Autodesk Inventor part; units mm, degrees
ref_plane "YZ Plane" through (0, 0, 0) normal (1, 0, 0) x (0, 1, 0)
ref_plane "XZ Plane" through (0, 0, 0) normal (0, 1, 0) x (-1, 0, 0)
ref_plane "XY Plane" through (0, 0, 0) normal (0, 0, 1) x (1, 0, 0)
sketch "スケッチ1" plane through (0, 0, 0) normal (1, 0, 0) x (0, 1, 0)
  line L0 (0, 0) -> (-96, 0)
  line L1 (-96, 0) -> (-96, -8)
  line L2 (-96, -8) -> (0, -8)
  line L3 (0, -8) -> (0, 0)
  line L4 (13, 5) -> (5, 5)
  line L5 (5, 5) -> (5, 75)
  line L6 (5, 75) -> (13, 75)
  line L7 (13, 75) -> (13, 5)
  line L8 (13, 5) -> (0, -8)
  line L9 (5, 5) -> (0, 0)
  line L10 (-44, 84) -> (13, 84)
  line L11 (13, 84) -> (13, 75)
  line L12 (-44, 76) -> (-44, 46)
  line L13 (-44, 46) -> (-36, 46)
  line L14 (-36, 46) -> (-36, 76)
  line L15 (5, 75) -> (5, 76)
  line L16 (5, 76) -> (-44, 76)
  line L17 (-44, 84) -> (-44, 76)
  point P0 (-36, 0)
  point P1 (-36, 76)
  point P2 (-44, 76)
  dimension "d0" = 8
  dimension "d2" = 8
  dimension "d3" = 70
  dimension "d4" = 96
  dimension "d17" = 13
  dimension "d36" = 8
  dimension "d37" = 41
  dimension "d53" = 1
  dimension "d54" = 8
  dimension "d55" = 30
  dimension "d72" = 57
  dimension "d86" = 30
extrude "押し出し1" add sketch "スケッチ1" along normal blind 80
sketch "スケッチ2" plane through (80, 0, 0) normal (1, 0, 0) x (0, 0, -1)
  line L0 (8, -96) -> (8, 0)
  point P0 (0, 0)
  point P1 (4, -71)
  point P2 (-50, 9)
  point P3 (-50, -40)
  dimension "d9" = 4
  dimension "d19" = 80
  dimension "d84" = 58
  dimension "d87" = 49
hole "穴1" at (80, -71, -4) at (80, 9, 50) at (80, -40, 50) direction (-1, 0, 0) diameter 2.459 depth 8.8 tip angle 118
sketch "スケッチ5" plane through (0, 13, 84) normal (0, 1, 0) x (1, 0, 0)
  line L0 (80, 8) -> (70, 8)
  line L1 (70, 8) -> (70, 30)
  line L2 (70, 30) -> (80, 30)
  line L3 (80, 30) -> (80, 8)
  line L4 (0, 0) -> (80, 0)
  line L5 (80, 79) -> (80, 0)
  point P0 (0, 84)
  dimension "d38" = 8
  dimension "d39" = 10
  dimension "d40" = 22
extrude "押し出し3" cut sketch "スケッチ5" against normal blind 80
sketch "スケッチ6" plane through (0, 13, 84) normal (0, 1, 0) x (1, 0, 0)
  line L0 (80, 8) -> (80, 0)
  line L1 (0, 0) -> (80, 0)
  point P0 (0, 84)
  point P1 (59.78, 12)
  point P2 (59.78, 26)
  dimension "d43" = 20.22
  dimension "d44" = 12
  dimension "d45" = 14
hole "穴3" at (59.78, 13, 72) at (59.78, 13, 58) direction (0, -1, 0) diameter 2.2 depth 8.8 tip angle 118
sketch "スケッチ7" plane through (0, -44, 46) normal (0, -1, 0) x (1, 0, 0)
  line L0 (80, 8) -> (80, 0)
  line L1 (80, 8) -> (70, 8)
  point P0 (0, -46)
  point P1 (67.7, 26.5)
  point P2 (67.7, 11.5)
  point P3 (52.7, 26.5)
  point P4 (52.7, 11.5)
  dimension "d58" = 15
  dimension "d59" = 15
  dimension "d60" = 12.3
  dimension "d61" = 3.5
hole "穴4" at (67.7, -44, 72.5) at (67.7, -44, 57.5) at (52.7, -44, 72.5) at (52.7, -44, 57.5) direction (0, 1, 0) diameter 2.2 depth 8 tip angle 118
sketch "スケッチ8" plane through (0, -44, 46) normal (0, -1, 0) x (1, 0, 0)
  line L0 (0, 38) -> (41.2, 38)
  line L1 (41.2, 38) -> (41.2, 8)
  line L2 (41.2, 8) -> (0, 8)
  line L3 (0, 8) -> (0, 38)
  line L4 (0, -46) -> (80, -46)
  line L5 (0, 38) -> (0, -46)
  line L6 (0, 38) -> (80, 38)
  circle A0 centre (52.7, 26.5) radius 1.1
  line L7 (80, 8) -> (70, 8)
  dimension "d75" = 11.5
  dimension "d83" = 0
extrude "押し出し4" cut sketch "スケッチ8" against normal blind 10 contours L0 L1 L2 L3
sketch "スケッチ9" plane through (0, -34, 46) normal (0, -1, 0) x (1, 0, 0)
  point P0 (0, -46)
sketch "スケッチ10" plane through (0, -34, 46) normal (0, -1, 0) x (1, 0, 0)
  line L0 (41.2, 38) -> (0, 38)
  line L1 (0, 38) -> (0, 30)
  line L2 (0, 30) -> (41.2, 30)
  line L3 (41.2, 30) -> (41.2, 38)
  line L4 (0, 38) -> (41.2, 38)
  line L5 (41.2, 38) -> (41.2, 8)
  line L6 (0, 30) -> (0, 38)
  line L7 (41.2, 30) -> (0, 30)
  point P0 (0, -46)
  point P1 (41.2, 0)
extrude "押し出し5" cut sketch "スケッチ10" against normal blind 39
sketch "スケッチ11" plane through (0, 5, 5) normal (0, -1, 0) x (1, 0, 0)
  point P0 (0, -5)
sketch "スケッチ12" plane through (0, 5, 5) normal (0, -1, 0) x (1, 0, 0)
  line L0 (41.2, 71) -> (49.2, 71)
  line L1 (49.2, 71) -> (49.2, 49)
  line L2 (49.2, 49) -> (41.2, 49)
  line L3 (41.2, 49) -> (41.2, 71)
  point P0 (0, -5)
  point P1 (70, 71)
  point P2 (41.2, 71)
  dimension "d76" = 8
  dimension "d77" = 22
extrude "押し出し6" add sketch "スケッチ12" along normal blind 49
sketch "スケッチ13" plane through (80, 0, 0) normal (1, 0, 0) x (0, 0, -1)
  line L0 (-54, 5) -> (-46, 5)
  line L1 (-46, 5) -> (-46, -36)
  line L2 (-46, -36) -> (-54, -36)
  line L3 (-54, -36) -> (-54, 5)
  line L4 (-54, 5) -> (-5, 5)
  line L5 (-46, -36) -> (-54, -36)
  line L6 (-54, 5) -> (-54, -36)
  line L7 (-46, -44) -> (-46, -36)
  point P0 (0, 0)
extrude "押し出し7" add sketch "スケッチ13" against normal blind 80
sketch "スケッチ14" plane through (0, 5, 46) normal (0, -1, 0) x (1, 0, 0)
  line L0 (70, -0.5) -> (20, -0.5)
  line L1 (20, -0.5) -> (20, -30.5)
  line L2 (20, -30.5) -> (70, -30.5)
  line L3 (70, -30.5) -> (70, -0.5)
  line L4 (0, -41) -> (0, 0)
  line L5 (0, 0) -> (80, 0)
  line L6 (64, -3.5) -> (26, -3.5)
  line L7 (26, -3.5) -> (26, -27.5)
  line L8 (26, -27.5) -> (64, -27.5)
  line L9 (64, -27.5) -> (64, -3.5)
  point P0 (0, -46)
  point P1 (0, -20.5)
  point P2 (67, -15.5)
  point P3 (23, -15.5)
  dimension "d88" = 20
  dimension "d89" = 30
  dimension "d90" = 50
  dimension "d91" = 0.5
  dimension "d92" = 6
  dimension "d93" = 6
  dimension "d94" = 3
  dimension "d95" = 3
  dimension "d98" = 44
  dimension "d99" = 3
extrude "押し出し8" cut sketch "スケッチ14" against normal blind 10 contours L9 L8 L7 L6
hole "穴5" at (67, 5, 30.5) at (23, 5, 30.5) direction (0, 1, 0) diameter 3.2 depth 8.8 tip angle 118
sketch "スケッチ15" plane through (0, -44, 46) normal (0, -1, 0) x (1, 0, 0)
  point P0 (0, -46)
sketch "スケッチ16" plane through (0, -44, 46) normal (0, -1, 0) x (1, 0, 0)
  line L0 (0, 0) -> (41.2, 0)
  line L1 (41.2, 0) -> (41.2, 8)
  line L2 (41.2, 8) -> (0, 8)
  line L3 (0, 8) -> (0, 0)
  point P0 (0, -46)
  dimension "d107" = 8
  dimension "d108" = 41.2
extrude "押し出し9" add sketch "スケッチ16" along normal blind 20
sketch "スケッチ20" plane through (0, 5, 54) normal (0, 0, 1) x (1, 0, 0)
  line L0 (15, -59) -> (23.5, -59)
  line L1 (23.5, -59) -> (23.5, -29)
  line L2 (23.5, -29) -> (15, -29)
  line L3 (15, -29) -> (15, -59)
  line L4 (41.2, -69) -> (0, -69)
  line L5 (0, -69) -> (0, 0)
  point P0 (0, -5)
  point P1 (19.25, -62.5)
  point P2 (19.25, -25.5)
  point P3 (23.5, -44)
  point P4 (19.25, -29)
  dimension "d111" = 10
  dimension "d112" = 30
  dimension "d113" = 37
  dimension "d114" = 8.5
  dimension "d115" = 15
  dimension "d116" = 18.5
extrude "押し出し10" cut sketch "スケッチ20" against normal blind 20
hole "穴6" at (19.25, -57.5, 54) at (19.25, -20.5, 54) direction (0, 0, -1) diameter 3.2 depth 8.8 tip angle 118
properties part number "左仕切り"
Read the model definition and answer for the solid it produces. Units are mm, in the model's axes. A direction names the side the tool comes from. Coordinates: 2 decimals unless noted, no trailing zeros. Write each loop counter-clockwise with the first axis right and the second up, starting at its lowest first coordinate (ties: lowest second). Pieces come first, ordered by that corner, then holes. Notation, with made-up numbers: (-16.5, 21) -> (38.5, 21) arc R15 ccw to (38.5, 26) -> close; hole circle Ø2 at (55, -7.5). An arc over 180 degrees is marked (long way). Write item = value, one per line.
(1) Section D-D on y = -57.5 is taken. Write down the section's boundary in (x, z).
From the geometry:
outline = (0, -8) -> (80, -8) -> (80, 0) -> (0, 0) -> close; (0, 46) -> (17.65, 46) -> (17.65, 54) -> (0, 54) -> close; (20.85, 46) -> (41.2, 46) -> (41.2, 54) -> (20.85, 54) -> close
(2) Section C-C on z = 24 is taken. Write down the section's boundary in (x, y), plus the area to 3 significant figures.
From the geometry:
outline = (0, 5) -> (26, 5) -> (26, 13) -> (0, 13) -> close; (64, 5) -> (80, 5) -> (80, 13) -> (64, 13) -> close
area = 336 mm2
(3) Which of the six approach directions +Z, -Z, +X, -X, +Y, -Y give full straight-line access (tool end or side, diameter ignored) to faces 4 (the face through (39, 5, 16)), 5 (the face through (75.54, -41.22, 50.16)), 6 (the face through (70, 9, 65)), 7 (the face through (19, -54, 50))?
From the geometry:
face_4 = +X, -X, -Y
face_5 = +X
face_6 = +X, +Y, -Y
face_7 = +Z
(4) Straight lines are drawn through the part: L1, parallel to X at y = -38, z = 72.5; L2, parallel to Z at x = 29, y = -37; L3, parallel to X at y = -57.5, z = 52. For each, find the intervals that lie inside material, in ascending order. Write a range as from..to.
From the geometry:
L1 = 41.2..51.6, 53.8..66.6, 68.8..70
L2 = -8..0, 46..54
L3 = 0..17.65, 20.85..41.2
(5) Section A-A on y = -10 is taken. Write down the section's boundary in (x, z).
From the geometry:
outline = (0, -8) -> (80, -8) -> (80, 0) -> (0, 0) -> close; (0, 46) -> (80, 46) -> (80, 54) -> (49.2, 54) -> (49.2, 76) -> (80, 76) -> (80, 84) -> (41.2, 84) -> (41.2, 54) -> (0, 54) -> close
(6) Section B-B on x = 38 is taken. Write down the section's boundary in (y, z), plus the area to 3 significant figures.
From the geometry:
outline = (-96, -8) -> (0, -8) -> (13, 5) -> (13, 18.5) -> (5, 18.5) -> (5, 5) -> (0, 0) -> (-96, 0) -> close; (-64, 46) -> (5, 46) -> (5, 42.5) -> (13, 42.5) -> (13, 84) -> (5, 84) -> (5, 54) -> (-64, 54) -> close
area = 1,830 mm2
(7) Given pin 1 Ø12 at (y, z) = (-41.5, 66) entering from +X; pin 2 Ø1 at (x, y) = (25, -37.5) entering from +Z; pin 3 Ø10 at (x, z) = (53, 39) entering from -Y; pin 4 Ø4 at (y, z) = (9, 50) entering from -X, each flat-ended and moving along its own axis, determine where each tip first touches the part or whether it passes through.
From the geometry:
pin_1 = 70
pin_2 = 54
pin_3 = 5
pin_4 = 0
(8) For a pull along Z with two mould halves and no side action, classify faces 1 (the face through (59, -36, 65)), 2 (the face through (39, 7, -1)), 3 (the face through (17.9, -58.36, 49.94)) as +Z half, -Z half, draft (parallel to the pull), parting line (faces both ways), or undercut.
From the geometry:
face_1 = undercut
face_2 = -Z half
face_3 = draft
